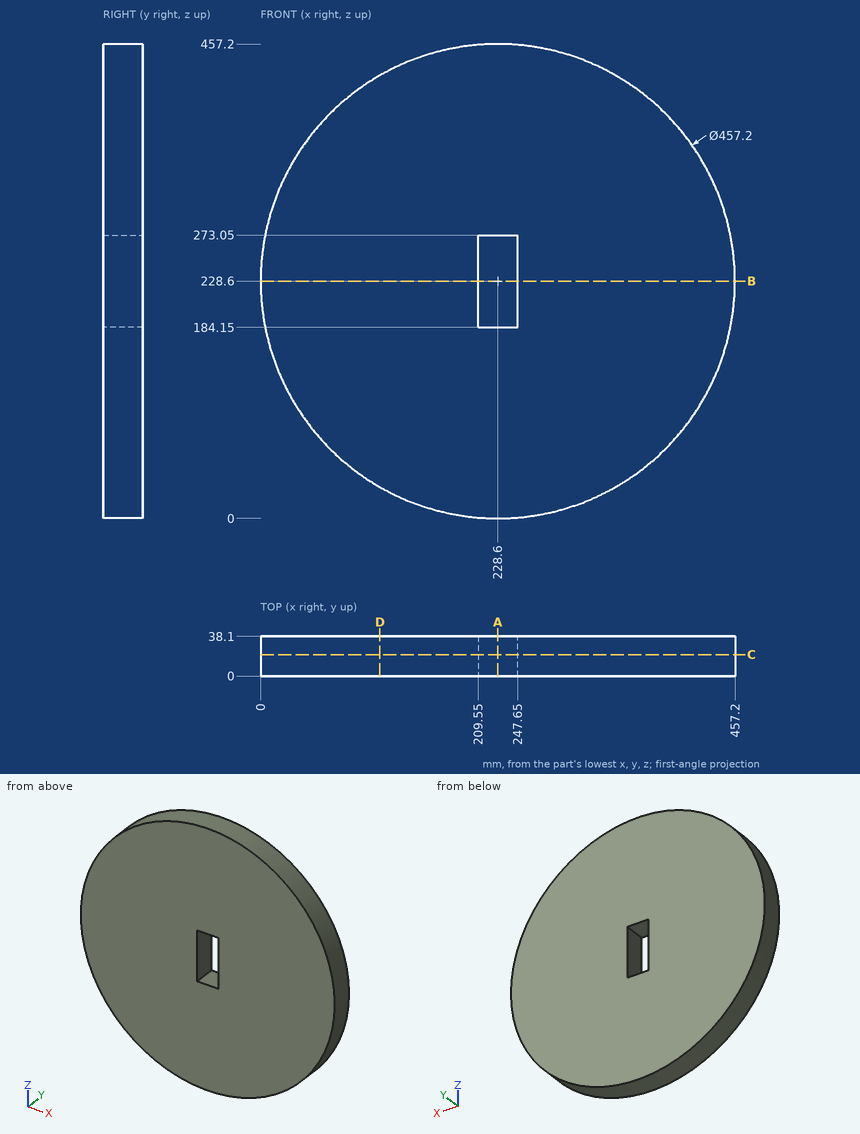
Verification items for this drawing (mm, ordinates from the low corner). Coordinates: 2 decimals unless noted, no trailing zeros. Order: outer loops, then holes, each group sorted by start corner. A loop starts at its lowest first (then second) coordinate and runs counter-clockwise, first axis right, second up. Notation, with made-up numbers: M 41.25,-4 L 87.25,-4 A27 cw 87.25,18 Z; hole C 31.5,79.5 d8. An arc over 180 degrees is marked long. Answer as a JSON object with one key per item and string values.
Q1. Cross-section at A-A on x = 228.6. Record the cut outline in (y, z), and give its area (3 significant figures).
Results are:
{"outline": "M 0,0 L 38.1,0 L 38.1,184.15 L 0,184.15 Z; M 0,273.05 L 38.1,273.05 L 38.1,457.2 L 0,457.2 Z", "area": "14,000 mm²"}
Q2. Scan lines: line 1 (X direction, y = 28.5, z = 231); line 2 (X direction, y = 31.5, z = 259.5); line 3 (Z direction, x = 243, y = 30.5). Record each from-to range of solid material in increasing order.
Results are:
{"line 1": "x = 0.01 to 209.55, 247.65 to 457.19", "line 2": "x = 2.1 to 209.55, 247.65 to 455.1", "line 3": "z = 0.45 to 184.15, 273.05 to 456.75"}
Q3. Cross-section at D-D on x = 115. Record the cut outline in (y, z).
Results are:
{"outline": "M 0,30.22 L 38.1,30.22 L 38.1,426.98 L 0,426.98 Z"}
Q4. Cross-section at B-B on z = 228.6. Record the cut outline in (x, y), and give its area (3 significant figures).
Results are:
{"outline": "M 0,0 L 209.55,0 L 209.55,38.1 L 0,38.1 Z; M 247.65,0 L 457.2,0 L 457.2,38.1 L 247.65,38.1 Z", "area": "16,000 mm²"}
Q5. Cross-section at C-C on y = 20.5. Record the cut outline in (x, z), and give its area (3 significant figures).
Results are:
{"outline": "C 228.6,228.6 d457.2; hole M 209.55,184.15 L 247.65,184.15 L 247.65,273.05 L 209.55,273.05 Z", "area": "161,000 mm²"}
Q6. Depth check by flat-ended pin: pin 1 Ø1 at (y, z) = (9.5, 277.5) entering from -X; pin 2 Ø4 at (x, z) = (301.5, 265) entering from -Y; pin 3 Ø1.5 at (x, y) = (271.5, 22.5) entering from -Z; pin 4 Ø1.5 at (y, z) = (29, 196.5) entering from -X. Enter the tip coordinate at first touch or a pass-through.
Results are:
{"pin 1": "stops at x = 5.18", "pin 2": "stops at y = 0", "pin 3": "stops at z = 3.92", "pin 4": "stops at x = 2.16"}
